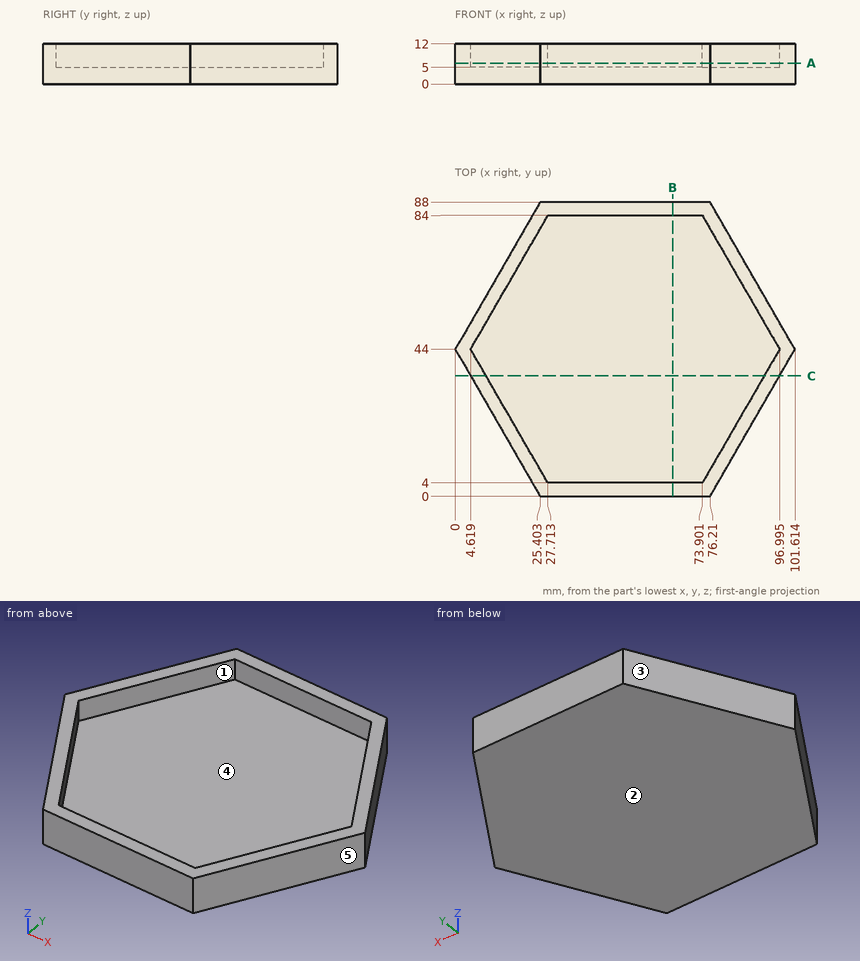
Geometry: see drawing. Coordinates: mm, zero at the bounding-box minimum. A direction names the side the tool comes from. Round coordinates to 2 decimals unless told otherwise and drop trailing zeros. Order: outer loops, then holes, each group sorted by start corner. A loop starts at its lowest first (then second) coordinate and runs counter-clockwise, first axis right, second up. Notation, with made-up numbers: (41, 64) - (55, 64) arc R15 ccw to (55, 80) - close; hole circle Ø1 at (44, 25). An arc over 180 degrees is marked (long way). Use a Markdown table: item, result. Add a question column.
1. Line query: probe 1 along Y at (x, z) = (59, 10.5); probe 2 along Z at (x, y) = (76, 46.5); probe 3 along X at (y, z) = (80, 8) (1 decimal). Output: solid intervals per line, ascending.
2. Section query C-C (y = 36). Return the cut outline in (x, z) (1 decimal).
3. Section query B-B (x = 65). Return the cut outline in (y, z), then the cut area to 3 significant figures.
4. First-contact query: pin 1 (5 mm diameter, centred on x = 72, y = 38.5, fed in from -Z); pin 2 (3 mm diameter, centred on x = 87.5, z = 2.5, fed in from -Y) (1 decimal); pin 3 (5 mm diameter, centred on x = 59, y = 18.5, fed in from +Z). Flat tips, straight axial feed; report the tip coordinate or a pass-through.
5. Set-up query: the marked faces 1 and 2. Return all of +Z, -Z, +X, -X, +Y, -Y with unobstructed straight access to the full face (end or side cutting, diameter ignored); none if empty.
6. Section query A-A (z = 6.25). Return the cut outline in (x, y) (1 decimal).
7. Mould query, pull axis X, two halves, no side actions, for the marked faces 3, 4 and 5. Classes: +X half, -X half, draft (parallel to the pull), parting line (faces both ways), or undercut.
Derived:
| question | item | result |
|---|---|---|
| 1 | probe 1 | 0 to 4, 84 to 88 |
| 1 | probe 2 | 0 to 5 |
| 1 | probe 3 | 20.8 to 25.4, 76.2 to 80.8 |
| 2 | outline | (4.6, 0) - (97, 0) - (97, 12) - (92.4, 12) - (92.4, 5) - (9.2, 5) - (9.2, 12) - (4.6, 12) - close |
| 3 | outline | (0, 0) - (88, 0) - (88, 12) - (84, 12) - (84, 5) - (4, 5) - (4, 12) - (0, 12) - close |
| 3 | area | 496 mm2 |
| 4 | pin 1 | z = 0 |
| 4 | pin 2 | y = 17 |
| 4 | pin 3 | z = 5 |
| 5 | face 1 | +Z |
| 5 | face 2 | -Z, +X, -X, +Y, -Y |
| 6 | outline | (0, 44) - (25.4, 0) - (76.2, 0) - (101.6, 44) - (76.2, 88) - (25.4, 88) - close; hole (4.6, 44) - (27.7, 4) - (73.9, 4) - (97, 44) - (73.9, 84) - (27.7, 84) - close |
| 7 | face 3 | -X half |
| 7 | face 4 | undercut |
| 7 | face 5 | +X half |
